Geometry check sheet. Reference: drawing and pictorial views, mm from the part's lowest x, y, z. Give positions to 0.01 mm unless a question says otherwise; leave off trailing zeros. Order: outer loops, then holes, each group sorted by start corner. A loop starts at its lowest first (then second) coordinate and runs counter-clockwise, first axis right, second up.
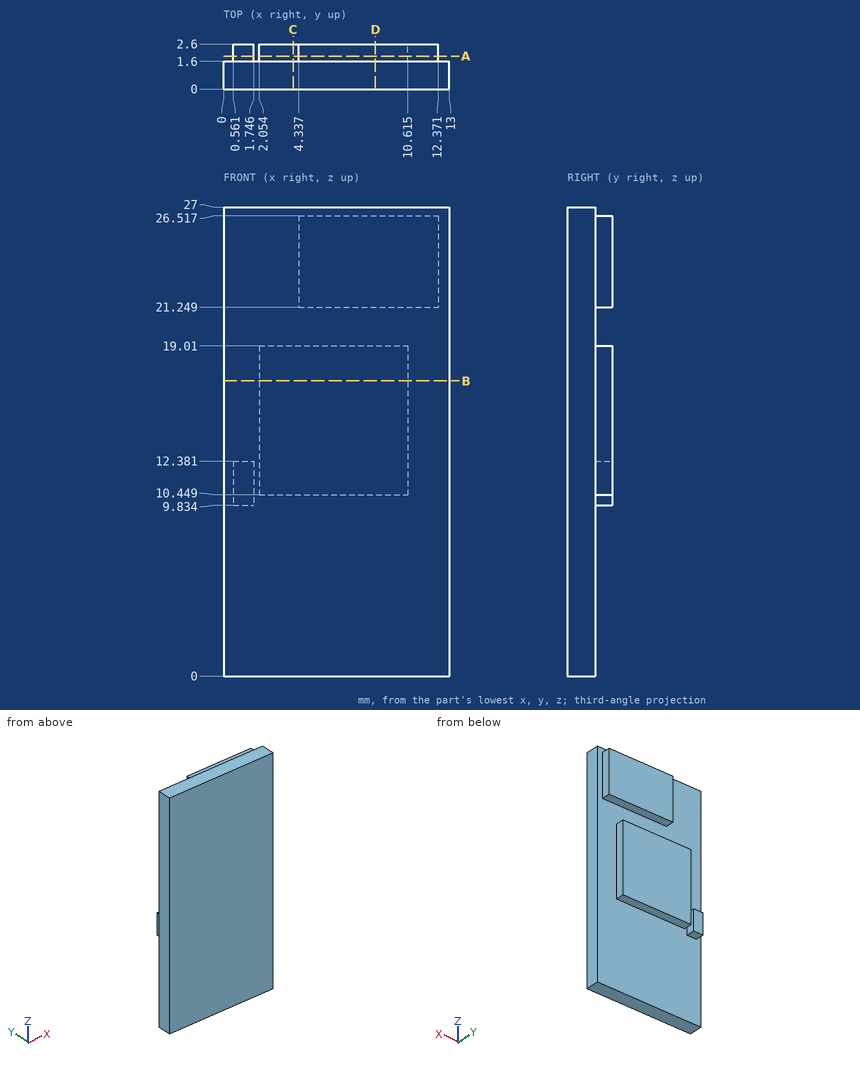
1) Section check C-C, the plane x = 4. Record the cut outline in (y, z).
Recorded:
outline: (0, 0) - (1.6, 0) - (1.6, 10.45) - (2.6, 10.45) - (2.6, 19.01) - (1.6, 19.01) - (1.6, 27) - (0, 27) - close
2) Depth check by flat-ended pin: pin 1 Ø1.1 at (y, z) = (2, 24.5) entering from -X; pin 2 Ø1.1 at (x, y) = (7, 2.5) entering from -Z; pin 3 Ø0.5 at (x, y) = (1, 2) entering from +Z; pin 4 Ø1 at (x, z) = (7.5, 8.5) entering from +Y. Enter the tip coordinate at first touch or a pass-through.
Recorded:
pin 1: stops at x = 0
pin 2: stops at z = 10.45
pin 3: stops at z = 12.38
pin 4: stops at y = 1.6
3) Material ranges on L1, parallel to Z at x = 8.25, y = 2.2; L2, parallel to X at y = 1.8, z = 16.75 (1 decimal); L3, parallel to Z at x = 1.5, y = 1.95 (1 decimal), recorded low to high.
Recorded:
L1: z = 10.45 to 19.01, 21.25 to 26.52
L2: x = 2.1 to 10.6
L3: z = 9.8 to 12.4
4) Section check B-B, the plane z = 17. Record the cut outline in (x, y) (1 decimal).
Recorded:
outline: (0, 0) - (13, 0) - (13, 1.6) - (10.6, 1.6) - (10.6, 2.6) - (2.1, 2.6) - (2.1, 1.6) - (0, 1.6) - close
5) Section check D-D, the plane x = 8.75. Record the cut outline in (y, z).
Recorded:
outline: (0, 0) - (1.6, 0) - (1.6, 10.45) - (2.6, 10.45) - (2.6, 19.01) - (1.6, 19.01) - (1.6, 21.25) - (2.6, 21.25) - (2.6, 26.52) - (1.6, 26.52) - (1.6, 27) - (0, 27) - close
6) Section check A-A, the plane y = 1.9. Record the cut outline in (x, z) (1 decimal).
Recorded:
outline: (0.6, 9.8) - (1.7, 9.8) - (1.7, 12.4) - (0.6, 12.4) - close; (2.1, 10.4) - (10.6, 10.4) - (10.6, 19) - (2.1, 19) - close; (4.3, 21.2) - (12.4, 21.2) - (12.4, 26.5) - (4.3, 26.5) - close
